Source: CAD feature listing. Evaluate the final solid. Frame: model axes, mm. A direction names the side the tool comes from. Round coordinates to 2 decimals unless told otherwise and drop trailing zeros. Loops run counter-clockwise (first coordinate to the right, second up) from the corner with the lowest first, then second, coordinate; pieces in that order, holes last. Notation, with made-up numbers: (7, 89.25) - (26, 89.25) arc R19 cw to (26, 108.25) - close; hole circle Ø7 at (35, -2.5). An arc over 180 degrees is marked (long way). One line per question, with ' | ' between items. Start each with the question number.
1. Cut plane A-A (z = 0). Return loops of the section in (x, y), then the cut area to 3 significant figures.
2. Cut plane B-B (x = 1). Return loops of the section in (y, z).
3. Pin query (flat end, axial travel): pin 1 (1.5 mm diameter, centred on x = 5.5, y = 147.5, fed in from +Z); pin 2 (13 mm diameter, centred on x = 0, z = 0, fed in from -Y); pin 3 (8 mm diameter, centred on y = -48, z = -6.5, fed in from +X). Return the tip coordinate at first contact, or that it passes through.
4. Access query for faces 1 (the cylindrical face through (-14.985, -4.41, 0.66)), 2 (the flat face through (0, -275, 0)), 3 (the flat face through (0, 275, 0)). Directions: +Z, -Z, +X, -X, +Y, -Y. A direction counts if a zero-diameter tool reaches every point of the face in a straight line with its end or side. Return the directions, or none.
5. Cut plane C-C (y = -246). Return loops of the section in (x, z).
6. Ray query, line 1 (Z direction, x = 0, y = -293); line 2 (Y direction, x = 2.75, z = -1.25); line 3 (Z direction, x = 1.25, y = -199). Return the intervals inside material, ascending.
```python
from build123d import *

# Parameters (mm, degrees)
F0_R     = 15
F1_DEPTH = 315
F2_R     = 7.25
F3_DEPTH = 40
F4_R     = 7.25
F5_DEPTH = 40


with BuildPart() as f1:
    # F0 (on Front) → F1 (new body, symmetric)
    with BuildSketch(Plane.XZ):
        Circle(F0_R)
    extrude(amount=F1_DEPTH, both=True)

    # F2 (on face) → F3 (cut)
    with BuildSketch(Plane.XZ.offset(315)):
        Circle(F2_R)
    extrude(amount=-F3_DEPTH, mode=Mode.SUBTRACT)

    # F4 (on face) → F5 (cut)
    with BuildSketch(Plane(origin=(0, 315, 0), x_dir=(-1, 0, 0), z_dir=(0, 1, 0))):
        Circle(F4_R)
    extrude(amount=-F5_DEPTH, mode=Mode.SUBTRACT)


solid = f1.part
```
Answers follow:
1) outline: (-15, -315) - (-7.25, -315) - (-7.25, -275) - (7.25, -275) - (7.25, -315) - (15, -315) - (15, 315) - (7.25, 315) - (7.25, 275) - (-7.25, 275) - (-7.25, 315) - (-15, 315) - close | area: 17,700 mm2
2) outline: (-315, -14.97) - (315, -14.97) - (315, -7.18) - (275, -7.18) - (275, 7.18) - (315, 7.18) - (315, 14.97) - (-315, 14.97) - (-315, 7.18) - (-275, 7.18) - (-275, -7.18) - (-315, -7.18) - close
3) pin 1: stops at z = 14.23 | pin 2: stops at y = -275 | pin 3: stops at x = 14.79
4) face 1: +Y, -Y | face 2: -Y | face 3: +Y
5) outline: circle Ø30 at (0, 0)
6) line 1: z = -15 to -7.25, 7.25 to 15 | line 2: y = -275 to 275 | line 3: z = -14.95 to 14.95
